Autodesk Inventor part; units mm, degrees
ref_plane "YZ Plane" through (0, 0, 0) normal (1, 0, 0) x (0, 1, 0)
ref_plane "XZ Plane" through (0, 0, 0) normal (0, 1, 0) x (-1, 0, 0)
ref_plane "XY Plane" through (0, 0, 0) normal (0, 0, 1) x (1, 0, 0)
sketch "Sketch1" plane through (0, 0, 0) normal (0, 0, 1) x (1, 0, 0)
  line L0 (-215, 140) -> (215, 140)
  line L1 (215, 140) -> (215, -140)
  line L2 (215, -140) -> (-215, -140)
  line L3 (-215, -140) -> (-215, 140)
  line L4 (-215, 140) -> (215, -140) construction
  line L5 (215, 140) -> (-215, -140) construction
  line L6 (0, 0) -> (0, -23) construction
  circle A0 centre (0, -23) radius 10
  dimension "d0" = 430
  dimension "d1" = 280
  dimension "d2" = 23
  dimension "d3" = 20
extrude "Extrusion1" add sketch "Sketch1" along normal blind 20
sketch "Sketch2" plane through (0, 0, 0) normal (0, 0, -1) x (-1, 0, 0)
  line L0 (215, -140) -> (-215, -140)
  line L1 (215, 140) -> (215, -140)
  line L2 (-215, 140) -> (215, 140)
  line L3 (-215, -140) -> (-215, 140)
  circle A0 centre (0, -23) radius 10
  line L4 (213, 138) -> (213, -138)
  line L5 (213, -138) -> (-213, -138)
  line L6 (-213, -138) -> (-213, 138)
  line L7 (-213, 138) -> (213, 138)
  point P0 (0, 0)
  dimension "d6" = 2
emboss "Emboss1" sketch "Sketch2" operation cut depth 1 direction (0, 0, 1) contours L4 L5 L6 L7
properties part number "SoporteBaseElevacion"
Here's how the part is built. I have some questions about the finished solid (model axes, mm). Give positions to 0.01 mm unless a question says otherwise; leave off trailing zeros. Write each loop counter-clockwise with the first axis right and the second up, starting at its lowest first coordinate (ties: lowest second). Pieces come first, ordered by that corner, then holes. Notation, with made-up numbers: (-32.5, -5.5) -> (0.5, -5.5) arc R20 cw to (0.5, 28.5) -> close; hole circle Ø6 at (49, -32). An arc over 180 degrees is marked (long way). Use one line per item in the form item = value.
1) I'm going to push flat-ended pins straight in: pin 1 (16 mm diameter, centred on x = 0, y = -23, fed in from -Z); pin 2 (8 mm diameter, centred on x = -58.5, y = -87.5, fed in from -Z). Where does each tip first touch, or does it pass through?
Verdict:
pin_1 = through
pin_2 = 1
2) If I drill on L1, parallel to X at y = -23, z = 8.5; L2, parallel to Y at x = 0, z = 9.25; L3, parallel to Z at x = -106, y = 100, over which ranges is the centre line in solid material (lowest first)? Write a range as [from, to].
Verdict:
L1 = [-215, -10], [10, 215]
L2 = [-140, -33], [-13, 140]
L3 = [1, 20]
3) Suppose I cut it at B-B (y = -23). Please give me the cut outline in (x, z).
Verdict:
outline = (-215, 0) -> (-213, 0) -> (-213, 1) -> (-10, 1) -> (-10, 20) -> (-215, 20) -> close; (10, 1) -> (213, 1) -> (213, 0) -> (215, 0) -> (215, 20) -> (10, 20) -> close
4) Suppose I cut it at A-A (x = 0). Please give me the cut outline in (y, z).
Verdict:
outline = (-140, 0) -> (-138, 0) -> (-138, 1) -> (-33, 1) -> (-33, 20) -> (-140, 20) -> close; (-13, 1) -> (138, 1) -> (138, 0) -> (140, 0) -> (140, 20) -> (-13, 20) -> close
5) We'd pull the mould along Y, two halves only. Please class faces 1 (the face through (3, -140, 10)), 2 (the face through (215, 2, 10)), 3 (the face through (-3, 2, 1)): +Y half, -Y half, draft (parallel to the pull), parting line (faces both ways), or undercut.
Verdict:
face_1 = -Y half
face_2 = draft
face_3 = undercut
6) Suppose I cut it at C-C (x = -183). Please give me the cut outline in (y, z), and give its area (3 significant figures).
Verdict:
outline = (-140, 0) -> (-138, 0) -> (-138, 1) -> (138, 1) -> (138, 0) -> (140, 0) -> (140, 20) -> (-140, 20) -> close
area = 5,320 mm2
